Source: CAD feature listing. Evaluate the final solid. Frame: model axes, mm. Face numbers are marked on the shaded views. A direction names the side the tool comes from. Give positions to 0.01 mm unless a question says otherwise; leave off trailing zeros. Order: outer loops, then holes, each group sorted by start corner. A loop starts at its lowest first (then second) coordinate and runs counter-clockwise, first axis right, second up.
from build123d import *

# Parameters (mm, degrees)
RESSALTO_EXTRUS_O1_DEPTH = 12.5
ESBO_O2_W                = 4
ESBO_O2_H                = 7
RESSALTO_EXTRUS_O2_DEPTH = 8.5
RESSALTO_EXTRUS_O3_DEPTH = 6
ESBO_O4_R                = 1.5
CORTE_EXTRUS_O1_DEPTH    = 6
FILETE1_R                = 6
CORTE_EXTRUS_O2_DEPTH    = 16.5


with BuildPart() as part:
    # Esboço1 → Ressalto-extrusão1 (new body)
    with BuildSketch(Plane.XY):
        Polygon((-9, 12.5), (9, 12.5), (14, 6.5), (14, -6.5), (-14, -6.5), (-14, 6.5), align=None)
    extrude(amount=RESSALTO_EXTRUS_O1_DEPTH)

    # Esboço2 → Ressalto-extrusão2 (add)
    with BuildSketch(Plane(origin=(0, 0, 0), x_dir=(-1, 0, 0), z_dir=(0, 0, -1))):
        with Locations((-7, 0)):
            Rectangle(ESBO_O2_W, ESBO_O2_H)
        with Locations((0, 6.5)):
            Rectangle(ESBO_O2_W, ESBO_O2_H)
        with Locations((7, 0)):
            Rectangle(ESBO_O2_W, ESBO_O2_H)
    extrude(amount=RESSALTO_EXTRUS_O2_DEPTH)

    # Esboço3 → Ressalto-extrusão3 (add)
    with BuildSketch(Plane.XY.offset(12.5)):
        Polygon((-9.5, -7.5), (9.5, -7.5), (32.25, 3), (9.5, 13.5), (-9.5, 13.5), (-32.25, 3), align=None)
    extrude(amount=RESSALTO_EXTRUS_O3_DEPTH)

    # Esboço4 → Corte-extrusão1 (cut)
    with BuildSketch(Plane.XY.offset(18.5)):
        with Locations((-20, 3)):
            Circle(ESBO_O4_R)
        with Locations((20, 3)):
            Circle(ESBO_O4_R)
    extrude(amount=-CORTE_EXTRUS_O1_DEPTH, mode=Mode.SUBTRACT)

    # Filete1
    filete1_edges = [part.edges().sort_by_distance(p)[0] for p in [
        (-32.25, 3, 15.5),
        (32.25, 3, 15.5),
    ]]
    fillet(filete1_edges, radius=FILETE1_R)

    # Esboço5 → Corte-extrusão2 (cut)
    with BuildSketch(Plane.XY.offset(18.5)):
        Polygon((-8, 12.404340661), (8, 12.404340661), (11.700014981, 8.793750875), (11.700014981, -2.595659339), (-11.299985019, -2.595659339), (-11.299985019, 8.404340661), align=None)
    extrude(amount=-CORTE_EXTRUS_O2_DEPTH, mode=Mode.SUBTRACT)


solid = part.part
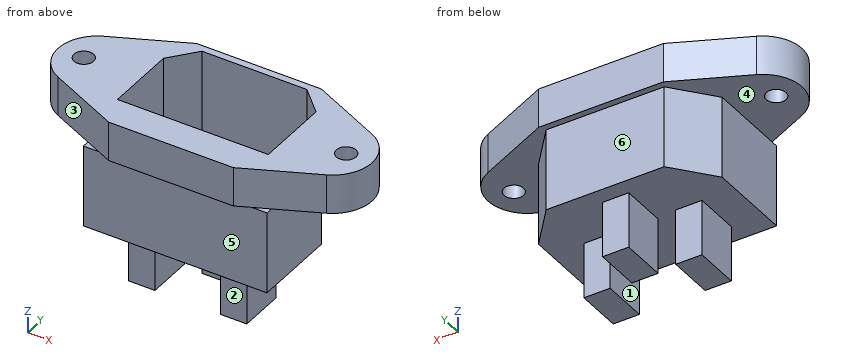
1) Section query D-D on x = 1.5. Output: boundary loops of the cut face in (y, z).
Checks:
outline: (-7.5, 12.5) - (-6.5, 12.5) - (-6.5, 0) - (3, 0) - (3, -8.5) - (10, -8.5) - (10, 0) - (12.5, 0) - (12.5, 12.5) - (13.5, 12.5) - (13.5, 18.5) - (12.4, 18.5) - (12.4, 2) - (-2.6, 2) - (-2.6, 18.5) - (-7.5, 18.5) - close
2) Section query A-A on z = -4.25. Output: boundary loops of the cut face in (x, y).
Checks:
outline: (-9, -3.5) - (-5, -3.5) - (-5, 3.5) - (-9, 3.5) - close; (-2, 3) - (2, 3) - (2, 10) - (-2, 10) - close; (5, -3.5) - (9, -3.5) - (9, 3.5) - (5, 3.5) - close
3) Ray query, L1, parallel to X at y = 2.5, z = 3.25; L2, parallel to Z at x = -16, y = -2.75; L3, parallel to Z at x = 11.5, y = -0.5. Return the intervals inside material, ascending.
Checks:
L1: x = -14 to -11.3, 11.7 to 14
L2: z = 12.5 to 18.5
L3: z = 0 to 2
4) Section query C-C on x = 19. Output: boundary loops of the cut face in (y, z), and give its area (3 significant figures).
Checks:
outline: (-3.12, 12.5) - (1.88, 12.5) - (1.88, 18.5) - (-3.12, 18.5) - close; (4.12, 12.5) - (9.12, 12.5) - (9.12, 18.5) - (4.12, 18.5) - close
area: 60.0 mm2
5) Section query B-B on z = 4.5. Output: boundary loops of the cut face in (x, y), and give its area (3 significant figures).
Checks:
outline: (-14, -6.5) - (14, -6.5) - (14, 6.5) - (9, 12.5) - (-9, 12.5) - (-14, 6.5) - close; hole (-11.3, -2.6) - (11.7, -2.6) - (11.7, 8.79) - (8, 12.4) - (-8, 12.4) - (-11.3, 8.4) - close
area: 170 mm2
6) Pull-direction query (X, two-part tool) for the marked faces 1, 2 and 3; classes: +X half, -X half, draft (parallel to the pull), parting line (faces both ways), or undercut.
Checks:
face 1: undercut
face 2: draft
face 3: -X half
7) Reachability of the marked faces 4, 5 and 6 from +Z, -Z, +X, -X, +Y, -Y: full face, straight path, thin tool, end or side. Return the list, or none.
Checks:
face 4: -Z, +Y
face 5: -Z, +X, -X, -Y
face 6: -Z, +X, -X, +Y
8) First-contact query: pin 1 Ø1.5 at (x, z) = (-4, 5.5) entering from -Y; pin 2 Ø3 at (y, z) = (7, 9.5) entering from -X; pin 3 Ø7.5 at (y, z) = (1, -3) entering from +X. Flat tips, straight axial feed; report the tip coordinate or a pass-through.
Checks:
pin 1: stops at y = -6.5
pin 2: stops at x = -14
pin 3: stops at x = 14
